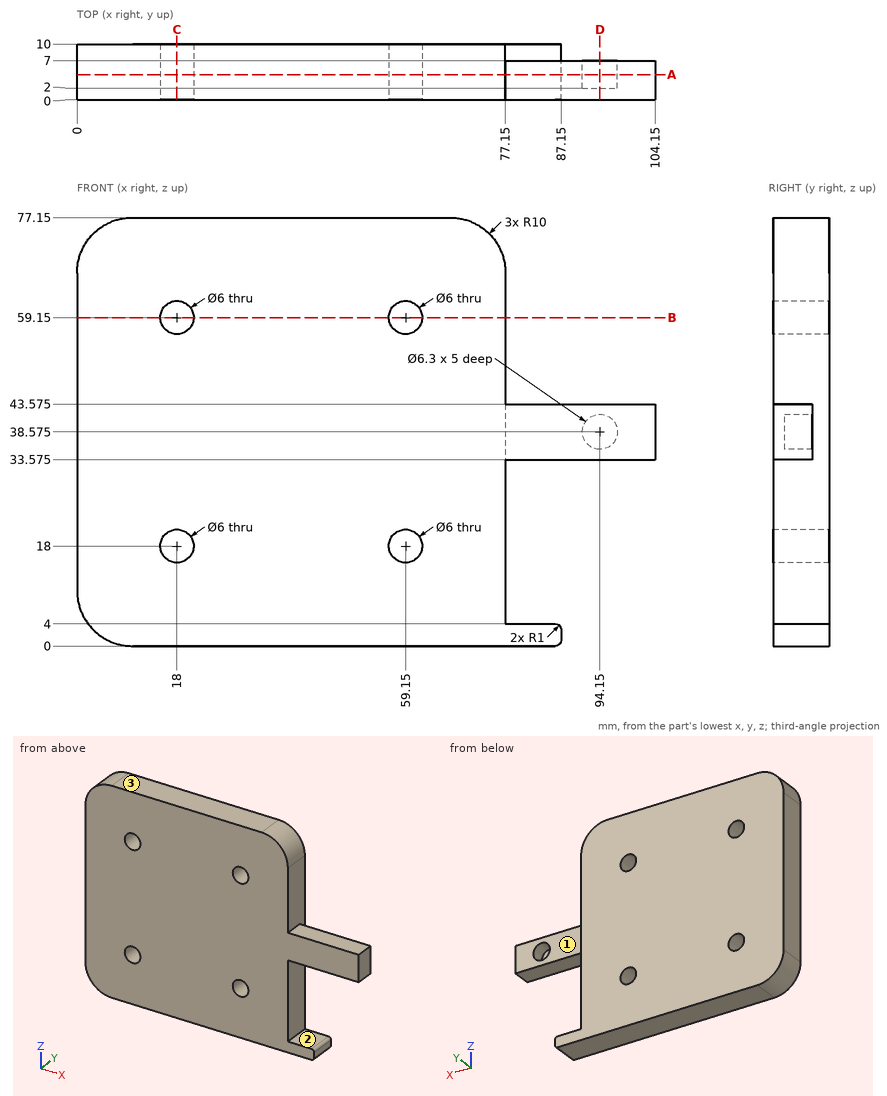
Geometry check sheet. Reference: drawing and pictorial views, mm from the part's lowest x, y, z. Give positions to 0.01 mm unless a question says otherwise; leave off trailing zeros. Order: outer loops, then holes, each group sorted by start corner. A loop starts at its lowest first (then second) coordinate and runs counter-clockwise, first axis right, second up. Notation, with made-up numbers: M -3,20 L 54,20 A5 cw 54,24 Z; hole C 41.25,66 d1. An arc over 180 degrees is marked long. Answer in a Markdown table with one row per item.
1) Cross-section at C-C, the plane x = 18. Enter the section's corners in (y, z).
Filled sheet:
| item | result |
|---|---|
| outline | M 0,0 L 10,0 L 10,15 L 0,15 Z; M 0,21 L 10,21 L 10,56.15 L 0,56.15 Z; M 0,62.15 L 10,62.15 L 10,77.15 L 0,77.15 Z |
2) Gauge pin test, flat ends, axial feed: P1, Ø2, axis at x = 75, y = 7, coming from the +Z side; P2, Ø1.9, axis at x = 94, z = 38, coming from the +Y side; P3, Ø11, axis at x = 91, z = 37, coming from the +Y side. Record the tip position at first contact, or that the pin passes through.
Filled sheet:
| item | result |
|---|---|
| P1 | stops at z = 74.44 |
| P2 | stops at y = 2 |
| P3 | stops at y = 7 |
3) Thickness scan on L1, parallel to X at y = 3.75, z = 59.15; L2, parallel to X at y = 3.25, z = 57; L3, parallel to Z at x = 97, y = 1.75 (3 decimals). Record the ranges inside material, lowest first. Write a range as [from, to].
Filled sheet:
| item | result |
|---|---|
| L1 | x = [0, 15], [21, 56.15], [62.15, 77.15] |
| L2 | x = [0, 15.91], [20.09, 57.06], [61.24, 77.15] |
| L3 | z = [33.575, 43.575] |
4) Cross-section at A-A, the plane y = 4.5. Enter the section's corners in (x, z) (3 decimals), plus the area to 3 significant figures.
Filled sheet:
| item | result |
|---|---|
| outline | M 0,10 A10 ccw 10,0 L 86.15,0 A1 ccw 87.15,1 L 87.15,3 A1 ccw 86.15,4 L 77.15,4 L 77.15,33.575 L 104.15,33.575 L 104.15,43.575 L 77.15,43.575 L 77.15,67.15 A10 ccw 67.15,77.15 L 10,77.15 A10 ccw 0,67.15 Z; hole C 18,18 d6; hole C 18,59.15 d6; hole C 59.15,18 d6; hole C 59.15,59.15 d6; hole C 94.15,38.575 d6.3 |
| area | 6,050 mm2 |
5) Cross-section at B-B, the plane z = 59.15. Enter the section's corners in (x, y).
Filled sheet:
| item | result |
|---|---|
| outline | M 0,0 L 15,0 L 15,10 L 0,10 Z; M 21,0 L 56.15,0 L 56.15,10 L 21,10 Z; M 62.15,0 L 77.15,0 L 77.15,10 L 62.15,10 Z |
6) Release check for a two-part mould opening along Z. For the marked faces 1, 2 and 3 record: +Z half, -Z half, draft (parallel to the pull), parting line (faces both ways), or undercut.
Filled sheet:
| item | result |
|---|---|
| face 1 | draft |
| face 2 | undercut |
| face 3 | +Z half |
7) Cross-section at D-D, the plane x = 94.15. Enter the section's corners in (y, z) (3 decimals).
Filled sheet:
| item | result |
|---|---|
| outline | M 0,33.575 L 7,33.575 L 7,35.425 L 2,35.425 L 2,41.725 L 7,41.725 L 7,43.575 L 0,43.575 Z |
